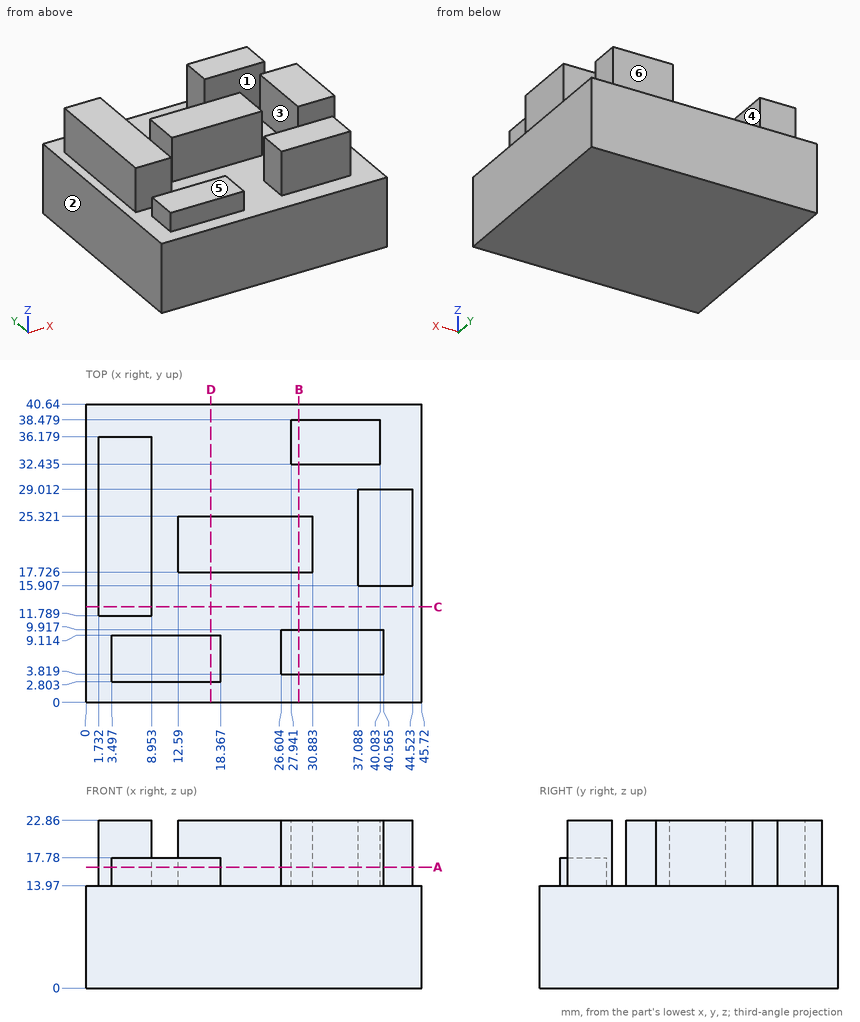
The figure shows three views and two pictorial views of one solid part (mm, origin at its lowest corner). Answer the questions. A direction names the side the tool comes from. Coordinates: 2 decimals unless noted, no trailing zeros. Write each loop counter-clockwise with the first axis right and the second up, starting at its lowest first coordinate (ties: lowest second). Pieces come first, ordered by that corner, then holes. Notation, with made-up numbers: (-14, 35) -> (31, 35) arc R29 cw to (31, 71) -> close; hole circle Ø10 at (19, 30.5). An arc over 180 degrees is marked (long way). Return JSON: item names as keys, results as strings.
1. Determine the mould class of the marked faces 1, 2 and 3 for opening direction X: pulls with the +X half, pulls with the -X half, needs draft (parallel to the pull), parting line crosses it, or undercut.
Found:
{"face 1": "needs draft", "face 2": "pulls with the -X half", "face 3": "undercut"}
2. A cutting plane is placed at D-D (x = 17). Determine the outline of the cut face in (y, z) (1 decimal).
Found:
{"outline": "(0, 0) -> (40.6, 0) -> (40.6, 14) -> (25.3, 14) -> (25.3, 22.9) -> (17.7, 22.9) -> (17.7, 14) -> (9.1, 14) -> (9.1, 17.8) -> (2.8, 17.8) -> (2.8, 14) -> (0, 14) -> close"}
3. A tool of negligible diameter and unlimited length cuts with its end or side. For the marked faces 4, 5 and 6, from which of +Z, -Z, +X, -X, +Y, -Y can it reach the whole face along a straight path? Write none if from no direction.
Found:
{"face 4": "+Z, +Y", "face 5": "+Z, -X, -Y", "face 6": "+Z, +X, -X, +Y"}
4. A cutting plane is placed at C-C (y = 13). Determine the outline of the cut face in (x, z), and give its area (3 significant figures).
Found:
{"outline": "(0, 0) -> (45.72, 0) -> (45.72, 13.97) -> (8.95, 13.97) -> (8.95, 22.86) -> (1.73, 22.86) -> (1.73, 13.97) -> (0, 13.97) -> close", "area": "703 mm2"}
5. A cutting plane is placed at B-B (x = 29). Determine the outline of the cut face in (y, z) (1 decimal).
Found:
{"outline": "(0, 0) -> (40.6, 0) -> (40.6, 14) -> (38.5, 14) -> (38.5, 22.9) -> (32.4, 22.9) -> (32.4, 14) -> (25.3, 14) -> (25.3, 22.9) -> (17.7, 22.9) -> (17.7, 14) -> (9.9, 14) -> (9.9, 22.9) -> (3.8, 22.9) -> (3.8, 14) -> (0, 14) -> close"}
6. Each of these flat-tipped pins is pushed along its axis until it touches: P1, Ø4.5, axis at x = 19.5, z = 17.5, coming from the +Y side; P2, Ø4.5, axis at x = 31.5, z = 19, coming from the -Y side; P3, Ø5, axis at x = 11, z = 18, coming from the -Y side. Where does it stop, or does it pass through?
Found:
{"P1": "y = 25.32", "P2": "y = 3.82", "P3": "y = 2.8"}
7. A cutting plane is placed at A-A (z = 16.5). Determine the outline of the cut face in (x, y) (1 decimal), and give its area (3 significant figures).
Found:
{"outline": "(1.7, 11.8) -> (9, 11.8) -> (9, 36.2) -> (1.7, 36.2) -> close; (3.5, 2.8) -> (18.4, 2.8) -> (18.4, 9.1) -> (3.5, 9.1) -> close; (12.6, 17.7) -> (30.9, 17.7) -> (30.9, 25.3) -> (12.6, 25.3) -> close; (26.6, 3.8) -> (40.6, 3.8) -> (40.6, 9.9) -> (26.6, 9.9) -> close; (27.9, 32.4) -> (40.1, 32.4) -> (40.1, 38.5) -> (27.9, 38.5) -> close; (37.1, 15.9) -> (44.5, 15.9) -> (44.5, 29) -> (37.1, 29) -> close", "area": "665 mm2"}
8. Find the intervals of material crossed by line 1 along X through (y, z) = (25, 21.25); line 2 along Y through (x, z) = (39, 22) (1 decimal); line 3 along Y through (x, z) = (5, 16) (1 decimal), in increasing order. Write a range as from..to.
Found:
{"line 1": "1.73..8.95, 12.59..30.88, 37.09..44.52", "line 2": "3.8..9.9, 15.9..29, 32.4..38.5", "line 3": "2.8..9.1, 11.8..36.2"}
